Here's how the part is built. I have some questions about the finished solid (model axes, mm). Coordinates: 2 decimals unless noted, no trailing zeros. Write each loop counter-clockwise with the first axis right and the second up, starting at its lowest first coordinate (ties: lowest second). Pieces come first, ordered by that corner, then holes. Notation, with made-up numbers: (-13.5, 49.5) - (30.5, 49.5) arc R22 ccw to (30.5, 77.5) - close; hole circle Ø6 at (81, 47). An arc over 180 degrees is marked (long way). Answer in a Markdown table with one row per item. Add a question column.
Item 1: I'm going to push flat-ended pins straight in: pin 1 (6 mm diameter, centred on y = 22, z = 119.5, fed in from +X); pin 2 (6 mm diameter, centred on y = -2.5, z = 49.5, fed in from +X); pin 3 (4 mm diameter, centred on y = -23, z = 116.5, fed in from -X); pin 4 (5 mm diameter, centred on x = -23, z = 194.5, fed in from +Y). Where does each tip first touch, or does it pass through?
Item 2: Imagine slicing it at C-C (z = 142). Please give me the cut outline in (x, y), plus the area to 3 significant figures.
Item 3: Imagine slicing it at A-A (y = 0). Please give me the cut outline in (x, z).
Item 4: If I drill on probe 1 along Y at (x, z) = (0, 90); probe 2 along Z at (x, y) = (9.5, 4); probe 3 along X at (y, z) = (12, 176), over which ranges is the centre line in solid material (lowest first)? Write a range as from..to.
Item 5: We'd pull the mould along X, two halves only. Please class faces 1 (the face through (0, 0, 2.54)), 2 (the face through (-24.08, -18.47, 109.88)), 3 (the face through (0, 0, 0)): +X half, -X half, draft (parallel to the pull), parting line (faces both ways), or undercut.
from build123d import *

# Parameters (mm, degrees)
F0_R     = 30.3497039052
F1_DEPTH = 220.726
F2_T     = -2.54


# Not quite as in the source:
# - a fillet or chamfer that OpenCascade refuses, or shapes differently, is made with other operations: its cross-section is extruded or revolved along the edge and cut away or added


with BuildPart() as f1:
    # F0 (on Top) → F1 (new body)
    with BuildSketch(Plane.XY):
        Circle(F0_R)
    extrude(amount=F1_DEPTH)

    # F2
    f2_openings = [f1.faces().sort_by_distance(p)[0] for p in [
        (0, 0, 220.726),
    ]]
    offset(amount=F2_T, openings=f2_openings)

    # F3: fillet of radius 7.62 on 3 edges, made by hand

    # F3_s1 → F3_t2 (revolve, cut)
    with BuildSketch(Plane.XZ):
        with BuildLine():
            ThreePointArc((30.3497039052, 7.62), (28.1178575778, 2.2318463274), (22.7297039052, 0))
            Line((22.7297039052, 0), (30.3497039052, 0))
            Line((30.3497039052, 0), (30.3497039052, 7.62))
        make_face()
    revolve(axis=Axis((0, 0, 0), (0, 0, 1)), mode=Mode.SUBTRACT)

    # F3_s3 → F3_t4 (revolve, cut)
    with BuildSketch(Plane.XZ):
        with BuildLine():
            ThreePointArc((30.3497039052, 215.0463873372), (29.6857803855, 218.1572393105), (27.8097039052, 220.726))
            Line((27.8097039052, 220.726), (30.3497039052, 220.726))
            Line((30.3497039052, 220.726), (30.3497039052, 215.0463873372))
        make_face()
    revolve(axis=Axis((0, 0, 220.726), (0, 0, 1)), mode=Mode.SUBTRACT)


solid = f1.part
Here are the results:
| question | item | result |
|---|---|---|
| 1 | pin 1 | stops at x = 23.67 |
| 1 | pin 2 | stops at x = 30.35 |
| 1 | pin 3 | stops at x = -21.91 |
| 1 | pin 4 | stops at y = 22.38 |
| 2 | outline | circle Ø60.7 at (0, 0); hole circle Ø55.62 at (0, 0) |
| 2 | area | 464 mm2 |
| 3 | outline | (-30.35, 7.62) arc R7.62 ccw to (-22.73, 0) - (22.73, 0) arc R7.62 ccw to (30.35, 7.62) - (30.35, 215.05) arc R7.62 ccw to (27.81, 220.73) - (27.81, 2.54) - (-27.81, 2.54) - (-27.81, 220.73) arc R7.62 ccw to (-30.35, 215.05) - close |
| 4 | probe 1 | y = -30.35..-27.81, 27.81..30.35 |
| 4 | probe 2 | z = 0..2.54 |
| 4 | probe 3 | x = -27.88..-25.09, 25.09..27.88 |
| 5 | face 1 | undercut |
| 5 | face 2 | parting line |
| 5 | face 3 | draft |
